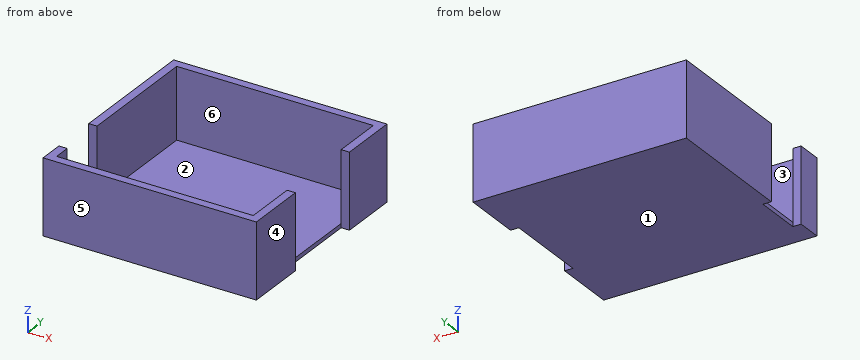
```python
from build123d import *

# Parameters (mm, degrees)
ESQUISSE1_W             = 51.2
ESQUISSE1_H             = 49.5
ESQUISSE1_W_2           = 47.2
ESQUISSE1_H_2           = 45.5
BOSS_EXTRU_1_DEPTH      = 17
ESQUISSE2_W             = 1
ESQUISSE2_H             = 49.5
BOSS_EXTRU_2_DEPTH      = 51.2
ESQUISSE3_W             = 2
ESQUISSE3_H             = 20.5
ESQUISSE3_H_2           = 11.3
ENL_V_MAT_EXTRU_2_DEPTH = 19


with BuildPart() as part:
    # Esquisse1 → Boss.-Extru.1 (new body)
    with BuildSketch(Plane.XY):
        with Locations((-0.122014971, -22.887662338)):
            Rectangle(ESQUISSE1_W, ESQUISSE1_H)
        with Locations((-0.122014971, -22.887662338)):
            Rectangle(ESQUISSE1_W_2, ESQUISSE1_H_2, mode=Mode.SUBTRACT)
    extrude(amount=BOSS_EXTRU_1_DEPTH)

    # Esquisse2 → Boss.-Extru.2 (add)
    with BuildSketch(Plane(origin=(25.477985029, 0, 0), x_dir=(0, 0, -1), z_dir=(1, 0, 0))):
        with Locations((0.5, -22.887662338)):
            Rectangle(ESQUISSE2_W, ESQUISSE2_H)
    extrude(amount=-BOSS_EXTRU_2_DEPTH)

    # Esquisse3 → Enlèv. mat.-Extru.2 (cut)
    with BuildSketch(Plane.XY.offset(17)):
        with Locations((24.477985029, -22.587662338)):
            Rectangle(ESQUISSE3_W, ESQUISSE3_H)
        with Locations((-24.722014971, -35.987662338)):
            Rectangle(ESQUISSE3_W, ESQUISSE3_H_2)
    extrude(amount=-ENL_V_MAT_EXTRU_2_DEPTH, mode=Mode.SUBTRACT)


solid = part.part
```
Part model, mm, in its own coordinate system. Face numbers are marked on the shaded views. A direction names the side the tool comes from. Round coordinates to 2 decimals unless told otherwise and drop trailing zeros. Loops run counter-clockwise (first coordinate to the right, second up) from the corner with the lowest first, then second, coordinate; pieces in that order, holes last. Notation, with made-up numbers: (-31.75, -26.75) -> (17.25, -26.75) arc R11 cw to (17.25, -21.75) -> close; hole circle Ø5 at (-17.75, 82). An arc over 180 degrees is marked (long way). Use a Markdown table: item, result.
1) Probe line 1 (X direction, y = -5, z = 0.75); line 2 (Y direction, x = 1, z = 2); line 3 (Z direction, x = 16.5, y = -1.5). List the from-to ranges inside material, lowest first. Write a range as [from, to].
The answers:
| item | result |
|---|---|
| line 1 | x = [-25.72, -23.72], [23.48, 25.48] |
| line 2 | y = [-47.64, -45.64], [-0.14, 1.86] |
| line 3 | z = [-1, 0] |
2) Drop flat-ended pins along their axis: pin 1 Ø0.5 at (y, z) = (-34, -0.5) entering from -X; pin 2 Ø8 at (x, y) = (12.5, -14) entering from +Z; pin 3 Ø1.5 at (y, z) = (-34.5, 10) entering from -X. Give the stop position or say it passes through.
The answers:
| item | result |
|---|---|
| pin 1 | stops at x = -23.72 |
| pin 2 | stops at z = 0 |
| pin 3 | stops at x = 23.48 |
3) Tool access for the marked faces 1 and 2: list every direction of +Z, -Z, +X, -X, +Y, -Y with a clear straight run to the whole face (end or side of a thin tool).
The answers:
| item | result |
|---|---|
| face 1 | -Z, +X, -X, +Y, -Y |
| face 2 | +Z |
4) Cut at A-A, the plane z = 7. List the corners of the cut face in (x, y).
The answers:
| item | result |
|---|---|
| outline | (-25.72, -47.64) -> (25.48, -47.64) -> (25.48, -32.84) -> (23.48, -32.84) -> (23.48, -45.64) -> (-23.72, -45.64) -> (-23.72, -41.64) -> (-25.72, -41.64) -> close; (-25.72, -30.34) -> (-23.72, -30.34) -> (-23.72, -0.14) -> (23.48, -0.14) -> (23.48, -12.34) -> (25.48, -12.34) -> (25.48, 1.86) -> (-25.72, 1.86) -> close |
5) Cut at C-C, the plane y = -23. List the corners of the cut face in (x, z).
The answers:
| item | result |
|---|---|
| outline | (-25.72, -1) -> (23.48, -1) -> (23.48, 0) -> (-23.72, 0) -> (-23.72, 17) -> (-25.72, 17) -> close |
6) Cut at B-B, the plane x = -18. List the corners of the cut face in (y, z).
The answers:
| item | result |
|---|---|
| outline | (-47.64, -1) -> (1.86, -1) -> (1.86, 17) -> (-0.14, 17) -> (-0.14, 0) -> (-45.64, 0) -> (-45.64, 17) -> (-47.64, 17) -> close |
7) Pull direction X, two halves, no side cores. Call the marked faces 3, 4, 5 and 6: pulls with the +X half, pulls with the -X half, needs draft (parallel to the pull), parting line crosses it, or undercut.
The answers:
| item | result |
|---|---|
| face 3 | undercut |
| face 4 | pulls with the +X half |
| face 5 | needs draft |
| face 6 | undercut |
